from build123d import *

# Parameters (mm, degrees)
EXTRUDE_1_DEPTH  = 13
EXTRUDE_2_DEPTH  = 3
EXTRUDE_3_DEPTH  = 15
FILLET_1_R       = 1
FILLET_2_R       = 1
FILLET_START     = -29.0000001
FILLET_3_DEPTH   = 29.0000001
FILLET_3_2_ANGLE = 180
FILLET_4_R       = 1
FILLET_5_R       = 1
FILLET_8_R       = 1


with BuildPart() as part:
    # 草图1 → 凸台-拉伸1 (new body)
    with BuildSketch(Plane.XY):
        with BuildLine():
            Line((-7.5, 114.244075086), (-12, 120.244075086))
            Line((-12, 120.244075086), (-15, 120.244075086))
            Line((-15, 120.244075086), (-15, 60.244075086))
            Line((-15, 60.244075086), (-12, 60.244075086))
            Line((-12, 60.244075086), (-7.5, 66.244075086))
            ThreePointArc((-7.5, 66.244075086), (-4.713203436, 77.469047246), (3, 86.087209919))
            Line((3, 86.087209919), (3, 94.400940253))
            ThreePointArc((3, 94.400940253), (-4.713203436, 103.019102925), (-7.5, 114.244075086))
        make_face()
    extrude(amount=EXTRUDE_1_DEPTH)

    # 草图3 → 凸台-拉伸2 (add)
    with BuildSketch(Plane(origin=(3, 0, 0), x_dir=(0, 0, -1), z_dir=(1, 0, 0))):
        with BuildLine():
            Line((1, 86.244075086), (-9, 86.244075086))
            ThreePointArc((-9, 86.244075086), (-13, 90.244075086), (-9, 94.244075086))
            Line((-9, 94.244075086), (1, 94.244075086))
            Line((1, 94.244075086), (15, 94.244075086))
            Line((15, 94.244075086), (25, 94.244075086))
            ThreePointArc((25, 94.244075086), (29, 90.244075086), (25, 86.244075086))
            Line((25, 86.244075086), (15, 86.244075086))
            Line((15, 86.244075086), (1, 86.244075086))
        make_face()
    extrude(amount=-EXTRUDE_2_DEPTH)

    # 草图4 → 凸台-拉伸3 (add)
    with BuildSketch(Plane.ZY):
        with BuildLine():
            Line((-15, 92.744075086), (-25, 92.744075086))
            ThreePointArc((-25, 92.744075086), (-27.5, 90.244075086), (-25, 87.744075086))
            Line((-25, 87.744075086), (-15, 87.744075086))
            ThreePointArc((-15, 87.744075086), (-12.5, 90.244075086), (-15, 92.744075086))
        make_face()
    extrude(amount=EXTRUDE_3_DEPTH)

    # 圆角1
    fillet_1_edges = [part.edges().sort_by_distance(p)[0] for p in [
        (3, 94.400940253, 6.5),
    ]]
    fillet(fillet_1_edges, radius=FILLET_1_R)

    # 圆角2
    fillet_2_edges = [part.edges().sort_by_distance(p)[0] for p in [
        (3, 86.087209919, 6.5),
    ]]
    fillet(fillet_2_edges, radius=FILLET_2_R)

    # 圆角3: read off the stored shape, not the designer's step
    # 圆角3 outline → 圆角3 (cut)
    with BuildSketch(Plane.XY.offset(FILLET_START)):
        with BuildLine():
            ThreePointArc((2, 94.244075086), (2.707106781, 93.951181867), (3, 93.244075086))
            Line((3, 93.244075086), (3, 93.878663231))
            ThreePointArc((3, 93.878663231), (2.9825594, 94.064612221), (2.930845947, 94.244075086))
            Line((2.930845947, 94.244075086), (2, 94.244075086))
        make_face()
        with BuildLine():
            Line((3, 86.60948694), (3, 87.244075086))
            ThreePointArc((3, 87.244075086), (2.707106781, 86.536968305), (2, 86.244075086))
            Line((2, 86.244075086), (2.930845947, 86.244075086))
            ThreePointArc((2.930845947, 86.244075086), (2.982559399, 86.423537951), (3, 86.60948694))
        make_face()
    extrude(amount=FILLET_3_DEPTH, mode=Mode.SUBTRACT)

    # Fillet 3 2 outline → Fillet 3 2 (revolve, cut)
    with BuildSketch(Plane(origin=(0, 90.244075086, -25), x_dir=(0, -1, 0), z_dir=(0, 0, 1))):
        with BuildLine():
            Line((4, 3), (3, 3))
            ThreePointArc((3, 3), (3.707106781, 2.707106781), (4, 2))
            Line((4, 2), (4, 3))
        make_face()
    revolve(axis=Axis((0, 90.244075086, -25), (1, 0, 0)), revolution_arc=FILLET_3_2_ANGLE, mode=Mode.SUBTRACT)

    # 圆角4
    fillet_4_edges = [part.edges().sort_by_distance(p)[0] for p in [
        (-12, 60.244075086, 6.5),
    ]]
    fillet(fillet_4_edges, radius=FILLET_4_R)

    # 圆角5
    fillet_5_edges = [part.edges().sort_by_distance(p)[0] for p in [
        (-12, 120.244075086, 6.5),
    ]]
    fillet(fillet_5_edges, radius=FILLET_5_R)

    # 圆角8
    fillet_8_edges = [part.edges().sort_by_distance(p)[0] for p in [
        (-7.5, 114.244075086, 6.5),
    ]]
    fillet(fillet_8_edges, radius=FILLET_8_R)


solid = part.part
Could you check a few things on this model? Use its own coordinates, in mm. A direction names the side the tool comes from. Round coordinates to 2 decimals unless told otherwise and drop trailing zeros. Write each loop counter-clockwise with the first axis right and the second up, starting at its lowest first coordinate (ties: lowest second). Pieces come first, ordered by that corner, then holes. Notation, with made-up numbers: (20.25, 5.5) - (43.25, 5.5) arc R28 cw to (43.25, 34.5) - close; hole circle Ø5 at (9.25, 84). An arc over 180 degrees is marked (long way). Use a Markdown table: item, result.
Q1. I want a section at D-D (z = -22). List the corners of the cut face in (x, y) for me.
Output values:
| item | result |
|---|---|
| outline | (-15, 87.74) - (0, 87.74) - (0, 86.24) - (2, 86.24) arc R1 ccw to (3, 87.24) - (3, 93.24) arc R1 ccw to (2, 94.24) - (0, 94.24) - (0, 92.74) - (-15, 92.74) - close |
Q2. For faces 1 (the flat face through (0, 90, -11)), 2 (the cylindrical face through (-7.4, 90.3, -27.5)), 3 (the flat face through (1, 86.244, -13)), 4 (the flat face through (-7, 87.744, -20)), which set-ups out of +Z, -Z, +X, -X, +Y, -Y let a thin tool reach every point of the face, with its end or its side?
Output values:
| item | result |
|---|---|
| face 1 | -X |
| face 2 | -Z, -X |
| face 3 | -Z, +X, -X, -Y |
| face 4 | -Z, -X, -Y |
Q3. For pin 1 (8 mm diameter, centred on x = -13, z = -23, fed in from -Y); pin 2 (2 mm diameter, centred on x = 1.5, z = -9.5, fed in from -Y); pin 3 (2 mm diameter, centred on y = 96.5, z = -6, fed in from -X); pin 4 (3 mm diameter, centred on x = -11.5, z = -13, fed in from +Y), each with a flat end and sliding along its axis, tell me the tip position at first contact or that it passes through.
Output values:
| item | result |
|---|---|
| pin 1 | y = 87.74 |
| pin 2 | y = 86.24 |
| pin 3 | through |
| pin 4 | y = 92.69 |
Q4. I want a section at B-B (z = 8). List the corners of the cut face in (x, y) for me.
Output values:
| item | result |
|---|---|
| outline | (-15, 60.24) - (-12.5, 60.24) arc R1 ccw to (-11.7, 60.64) - (-7.5, 66.24) arc R24 cw to (2.58, 85.79) arc R1 ccw to (3, 86.61) - (3, 93.88) arc R1 ccw to (2.58, 94.69) arc R24 cw to (-7.5, 113.92) arc R1 ccw to (-7.7, 114.51) - (-11.7, 119.84) arc R1 ccw to (-12.5, 120.24) - (-15, 120.24) - close |
Q5. I want a section at A-A (x = -10). List the corners of the cut face in (y, z) for me, plus the area to 3 significant figures.
Output values:
| item | result |
|---|---|
| outline | (62.91, 0) - (117.58, 0) - (117.58, 13) - (62.91, 13) - close; (87.74, -25) arc R2.5 ccw to (92.74, -25) - (92.74, -15) arc R2.5 ccw to (87.74, -15) - close |
| area | 780 mm2 |
Q6. Please list where these lines run through material, in increasing order: L1, parallel to Z at x = -5, y = 90; L2, parallel to Z at x = -7, y = 78; L3, parallel to Y at x = -0.25, z = -24.
Output values:
| item | result |
|---|---|
| L1 | -27.49 to -12.51, 0 to 13 |
| L2 | 0 to 13 |
| L3 | 87.74 to 92.74 |
Q7. Thinking about a two-plate mould opening in Z: for faces 5 (the flat face through (-7, 92.744, -20)), 6 (the flat face through (-8, 91, 13)), 7 (the flat face through (-10, 91, 0)), which applies, released by +Z, released by -Z, zero draft, split by the parting line, or undercut?
Output values:
| item | result |
|---|---|
| face 5 | zero draft |
| face 6 | released by +Z |
| face 7 | undercut |
Q8. I want a section at C-C (y = 96). List the corners of the cut face in (x, z) for me, plus the area to 3 significant figures.
Output values:
| item | result |
|---|---|
| outline | (-15, 0) - (0.91, 0) - (0.91, 13) - (-15, 13) - close |
| area | 207 mm2 |
